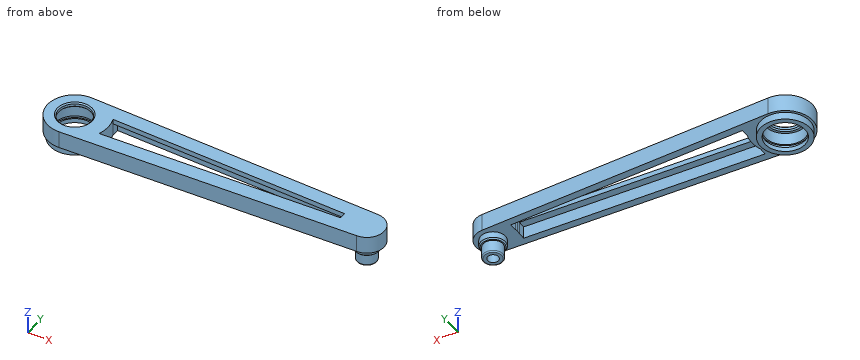
```python
from build123d import *

# Parameters (mm, degrees)
SKETCH_1_R          = 8.075
EXTRUDE_1_DEPTH     = 7
EXTRUDE_START       = -2
SKETCH_2_R          = 8.075
SKETCH_2_R_2        = 6.575
EXTRUDE_2_DEPTH     = 2
SKETCH_3_R          = 4
EXTRUDE_3_DEPTH     = 10
SKETCH_4_R          = 5
SKETCH_4_R_2        = 4
EXTRUDE_4_DEPTH     = 3
CHAMFER_1_SIZE      = 0.5
CUT_EXTRUDE_1_DEPTH = 7
CUT_EXTRUDE_2_DEPTH = 5
CUT_EXTRUDE_START   = -2
SKETCH_8_R          = 4
CUT_EXTRUDE_3_DEPTH = 2
FILLET_1_R          = 0.5
SKETCH_9_R          = 2.2
CUT_EXTRUDE_4_DEPTH = 10
EXTRUDE_START_2     = 3
SKETCH_10_R         = 10.075
SKETCH_10_R_2       = 8.075
EXTRUDE_5_DEPTH     = 3


with BuildPart() as part:
    # 草图1 → 凸台-拉伸1 (new body)
    with BuildSketch(Plane.XY):
        with BuildLine():
            ThreePointArc((0.37924895, 11.068504652), (-11.074999998, -0.000191538), (0.379631801, -11.068491528))
            Line((0.379631801, -11.068491528), (119, -7))
            ThreePointArc((119, -7), (125.998973572, -0.119870518), (119.239705882, 6.995894588))
            Line((119.239705882, 6.995894588), (0.37924895, 11.068504652))
        make_face()
        Circle(SKETCH_1_R, mode=Mode.SUBTRACT)
    extrude(amount=EXTRUDE_1_DEPTH)

    # 草图2 → 凸台-拉伸2 (add)
    with BuildSketch(Plane.XY.offset(7).offset(EXTRUDE_START)):
        Circle(SKETCH_2_R)
        Circle(SKETCH_2_R_2, mode=Mode.SUBTRACT)
    extrude(amount=EXTRUDE_2_DEPTH)

    # 草图3 → 凸台-拉伸3 (add)
    with BuildSketch(Plane(origin=(0, 0, 0), x_dir=(-1, 0, 0), z_dir=(0, 0, -1))):
        with Locations((-119, 0)):
            Circle(SKETCH_3_R)
    extrude(amount=EXTRUDE_3_DEPTH)

    # 草图4 → 凸台-拉伸4 (add)
    with BuildSketch(Plane(origin=(0, 0, 0), x_dir=(-1, 0, 0), z_dir=(0, 0, -1))):
        with Locations(Location((-119, 0, 0), (0, 0, 180))):
            Circle(SKETCH_4_R)
        with Locations((-119, 0)):
            Circle(SKETCH_4_R_2, mode=Mode.SUBTRACT)
    extrude(amount=EXTRUDE_4_DEPTH)

    # 倒角1
    chamfer_1_edges = [part.edges().sort_by_distance(p)[0] for p in [
        (-6.575, 0, 5),
        (-6.575, 0, 7),
        (123, 0, -10),
        (114, 0, -3),
    ]]
    chamfer(chamfer_1_edges, length=CHAMFER_1_SIZE)

    # 草图5 → 切除-拉伸1 (cut)
    with BuildSketch(Plane(origin=(0, 0, 0), x_dir=(-1, 0, 0), z_dir=(0, 0, -1))):
        with BuildLine():
            ThreePointArc((-12.757234161, -4.640431182), (-13.574999998, 0.000234775), (-12.757073645, 4.640872443))
            Line((-12.757073645, 4.640872443), (-109.090204802, 1.340134001))
            ThreePointArc((-109.090204802, 1.340134001), (-109.022576686, 0.671583213), (-109, 0))
            ThreePointArc((-109, 0), (-109.022449652, -0.669693251), (-109.08969781, -1.336379625))
            Line((-109.08969781, -1.336379625), (-12.757234161, -4.640431182))
        make_face()
    extrude(amount=-CUT_EXTRUDE_1_DEPTH, mode=Mode.SUBTRACT)

    # 草图6 → 切除-拉伸2 (cut)
    with BuildSketch(Plane(origin=(0, 0, 0), x_dir=(-1, 0, 0), z_dir=(0, 0, -1))):
        Polygon((-109.08969781, -1.336379625), (-12.757234161, -4.640431182), (-12.860068961, -7.638668165), (-109.192532609, -4.334616608), align=None)
        Polygon((-12.757073645, 4.640872443), (-109.090204802, 1.340134001), (-109.192935895, 4.338374538), (-12.859804737, 7.63911298), align=None)
    extrude(amount=-CUT_EXTRUDE_2_DEPTH, mode=Mode.SUBTRACT)

    # 草图8 → 切除-拉伸3 (cut)
    with BuildSketch(Plane(origin=(0, 0, -10), x_dir=(-1, 0, 0), z_dir=(0, 0, -1)).offset(CUT_EXTRUDE_START)):
        with Locations((-119, 0)):
            Circle(SKETCH_8_R)
    extrude(amount=CUT_EXTRUDE_3_DEPTH, mode=Mode.SUBTRACT)

    # 圆角1
    fillet_1_edges = [part.edges().sort_by_distance(p)[0] for p in [
        (123, 0, -8),
    ]]
    fillet(fillet_1_edges, radius=FILLET_1_R)

    # 草图9 → 切除-拉伸4 (cut)
    with BuildSketch(Plane(origin=(0, 0, -8), x_dir=(-1, 0, 0), z_dir=(0, 0, -1))):
        with Locations((-119, 0)):
            Circle(SKETCH_9_R)
    extrude(amount=-CUT_EXTRUDE_4_DEPTH, mode=Mode.SUBTRACT)

    # 草图10 → 凸台-拉伸5 (add)
    with BuildSketch(Plane(origin=(0, 0, 0), x_dir=(-1, 0, 0), z_dir=(0, 0, -1)).offset(EXTRUDE_START_2)):
        with Locations(Location((0, 0, 0), (0, 0, 180))):
            Circle(SKETCH_10_R)
        Circle(SKETCH_10_R_2, mode=Mode.SUBTRACT)
    extrude(amount=-EXTRUDE_5_DEPTH)

    # 切除-旋转2: read off the stored shape, not the designer's step
    # 切除-旋转2: loft between two sections, ruled curve by curve
    cut_revolve_2_from = [
        Edge.make_three_point_arc((8.65, 0, -1.2), (0, 8.65, -1.2), (-8.65, 0, -1.2)),
        Edge.make_three_point_arc((-8.65, 0, -1.2), (0, -8.65, -1.2), (8.65, 0, -1.2)),
    ]
    cut_revolve_2_to = [
        Edge.make_three_point_arc((8.65, 0, 0), (0, 8.65, 0), (-8.65, 0, 0)),
        Edge.make_three_point_arc((-8.65, 0, 0), (0, -8.65, 0), (8.65, 0, 0)),
    ]
    cut_revolve_2 = Solid(Shell([*[Face.make_surface_from_curves(cut_revolve_2_from[k], cut_revolve_2_to[k]) for k in range(2)], Face(Wire(cut_revolve_2_from)), Face(Wire(cut_revolve_2_to))]))
    add(cut_revolve_2, mode=Mode.SUBTRACT)


solid = part.part
```
Here's how the part is built. I have some questions about the finished solid (model axes, mm). Coordinates: 2 decimals unless noted, no trailing zeros. Order: outer loops, then holes, each group sorted by start corner. A loop starts at its lowest first (then second) coordinate and runs counter-clockwise, first axis right, second up. Notation, with made-up numbers: (37, 20) -> (94, 20) arc R13 ccw to (94, 41) -> close; hole circle Ø3 at (-37, 69). An arc over 180 degrees is marked (long way). Return JSON: item names as keys, results as strings.
1) I'm going to push flat-ended pins straight in: P1, Ø13, axis at x = 0, y = 0, coming from the +Z side; P2, Ø1, axis at y = -4.5, z = 3.5, coming from the +X side; P3, Ø4, axis at x = 88, z = 2.5, coming from the -Y side; P4, Ø8, axis at x = 66, y = -8.5, coming from the -Z side. Where does each tip first touch, or does it pass through?
Conclusion:
{"P1": "passes through", "P2": "stops at x = 124.74", "P3": "stops at y = -8.13", "P4": "stops at z = 0"}
2) If we section it at A-A on x = 41: List the corners of the cut face in (y, z) for me.
Conclusion:
{"outline": "(-9.68, 0) -> (-6.67, 0) -> (-6.67, 5) -> (-3.67, 5) -> (-3.67, 7) -> (-9.68, 7) -> close; (3.67, 5) -> (6.67, 5) -> (6.67, 0) -> (9.68, 0) -> (9.68, 7) -> (3.67, 7) -> close"}
3) If I drill on probe 1 along Y at (x, z) = (119, -4.5); probe 2 along Y at (x, z) = (0, 6.2) (3 decimals); probe 3 along X at (y, z) = (1, 2.5), over which ranges is the centre line in solid material (lowest first)?
Conclusion:
{"probe 1": "y = -4 to -2.2, 2.2 to 4", "probe 2": "y = -11.075 to -6.575, 6.575 to 11.075", "probe 3": "x = -11.03 to -8.01, 8.01 to 13.54, 109.05 to 125.93"}
